For this review, use the dimensioned drawing (mm, ordinates from the lowest corner) and the shaded views. A direction names the side the tool comes from. Round coordinates to 2 decimals unless told otherwise and drop trailing zeros. Loops run counter-clockwise (first coordinate to the right, second up) from the corner with the lowest first, then second, coordinate; pieces in that order, holes last. Notation, with made-up numbers: (7, 34) -> (40, 34) arc R22 cw to (40, 46) -> close; hole circle Ø9 at (-3.5, -16.5). An arc over 180 degrees is marked (long way). Write each question's results on one line, items separated by ' | '.
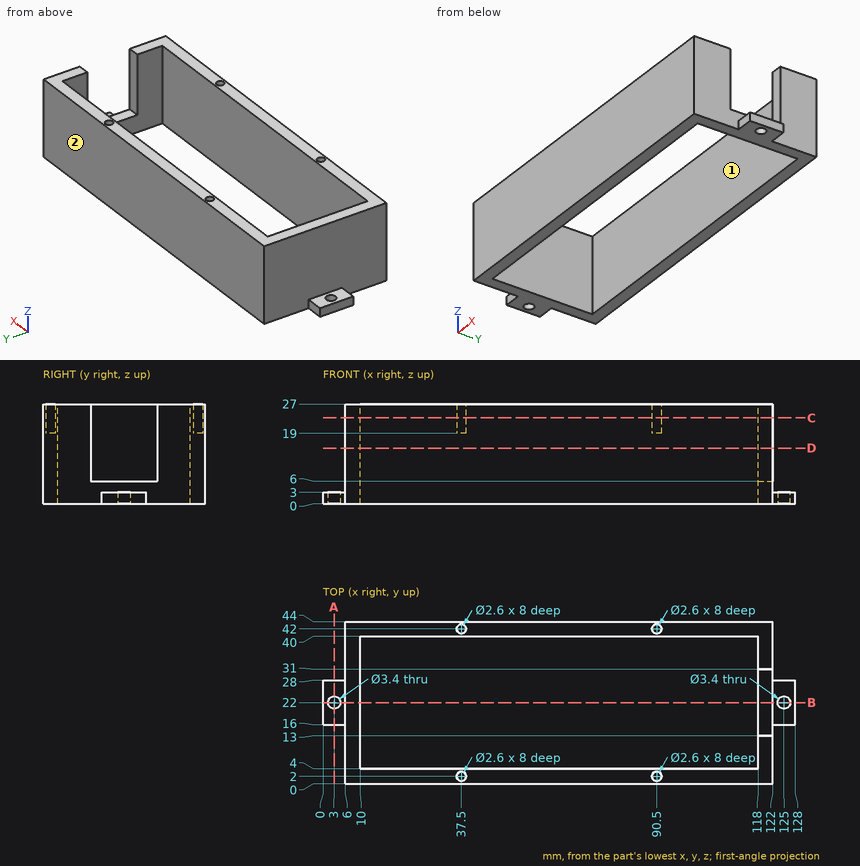
1. Consider section B-B (y = 22). State the section outline as (x, z) points.
Values found:
outline: (0, 0) -> (1.3, 0) -> (1.3, 3) -> (0, 3) -> close; (4.7, 0) -> (10, 0) -> (10, 27) -> (6, 27) -> (6, 3) -> (4.7, 3) -> close; (118, 0) -> (123.3, 0) -> (123.3, 3) -> (122, 3) -> (122, 6) -> (118, 6) -> close; (126.7, 0) -> (128, 0) -> (128, 3) -> (126.7, 3) -> close
2. Tool access review of the marked faces 1 and 2: name each direction out of +Z, -Z, +X, -X, +Y, -Y from which nothing blocks a thin tool from reaching the whole face with its end or side.
Values found:
face 1: +Z, -Z | face 2: +Z, -Z, +X, -X, +Y
3. To check wall thickness, follow probe 1 along X at (y, z) = (42, 23.5); probe 2 along Y at (x, z) = (37.5, 22.75); probe 3 along X at (y, z) = (22, 2.3). State the ranges of each line that lie inside material, in increasing order.
Values found:
probe 1: x = 6 to 36.2, 38.8 to 89.2, 91.8 to 122 | probe 2: y = 0 to 0.7, 3.3 to 4, 40 to 40.7, 43.3 to 44 | probe 3: x = 0 to 1.3, 4.7 to 10, 118 to 123.3, 126.7 to 128
4. Consider section D-D (z = 15). State the section outline as (x, y) points.
Values found:
outline: (6, 0) -> (122, 0) -> (122, 13) -> (118, 13) -> (118, 4) -> (10, 4) -> (10, 40) -> (118, 40) -> (118, 31) -> (122, 31) -> (122, 44) -> (6, 44) -> close
5. Consider section A-A (x = 3). State the section outline as (y, z) points.
Values found:
outline: (16, 0) -> (20.3, 0) -> (20.3, 3) -> (16, 3) -> close; (23.7, 0) -> (28, 0) -> (28, 3) -> (23.7, 3) -> close
6. Consider section C-C (z = 23.25). State the section outline as (x, y) points.
Values found:
outline: (6, 0) -> (122, 0) -> (122, 13) -> (118, 13) -> (118, 4) -> (10, 4) -> (10, 40) -> (118, 40) -> (118, 31) -> (122, 31) -> (122, 44) -> (6, 44) -> close; hole circle Ø2.6 at (37.5, 2); hole circle Ø2.6 at (37.5, 42); hole circle Ø2.6 at (90.5, 2); hole circle Ø2.6 at (90.5, 42)
7. For pin 1 (1.6 mm diameter, centred on x = 90.5, y = 42, fed in from +Z); pin 2 (3.5 mm diameter, centred on x = 3, z = 1.5, fed in from +Y); pin 3 (8 mm diameter, centred on y = 32.5, z = 18.5, fed in from -X), all flat-tipped, find the tip position at first contact; note any pin that passes through.
Values found:
pin 1: stops at z = 19 | pin 2: stops at y = 28 | pin 3: stops at x = 6
